Study the drawing (mm; zero at the part's minimum x, y, z) and answer. Coordinates: 2 decimals unless noted, no trailing zeros. Order: outer loops, then holes, each group sorted by start corner. A loop starts at its lowest first (then second) coordinate and runs counter-clockwise, first axis right, second up. Notation, with made-up numbers: M 71.25,82.5 L 93.25,82.5 A29 ccw 93.25,108.5 Z; hole C -33.5,12.5 d2. An arc over 180 degrees is marked long. Use a Markdown table: item, result. Add a question column.
1) Find the intervals of material crossed by probe 1 along Y at (x, z) = (85.5, 2); probe 2 along Y at (x, z) = (96, 1.8), in increasing order. Write a range as [from, to].
2) Find section B-B on z = 3.25. Count the separate pieces of the cut face and the enclosed holes in it, plus the area to 3 significant figures.
3) Find section A-A on x = 154. Write down the section's boundary in (y, z).
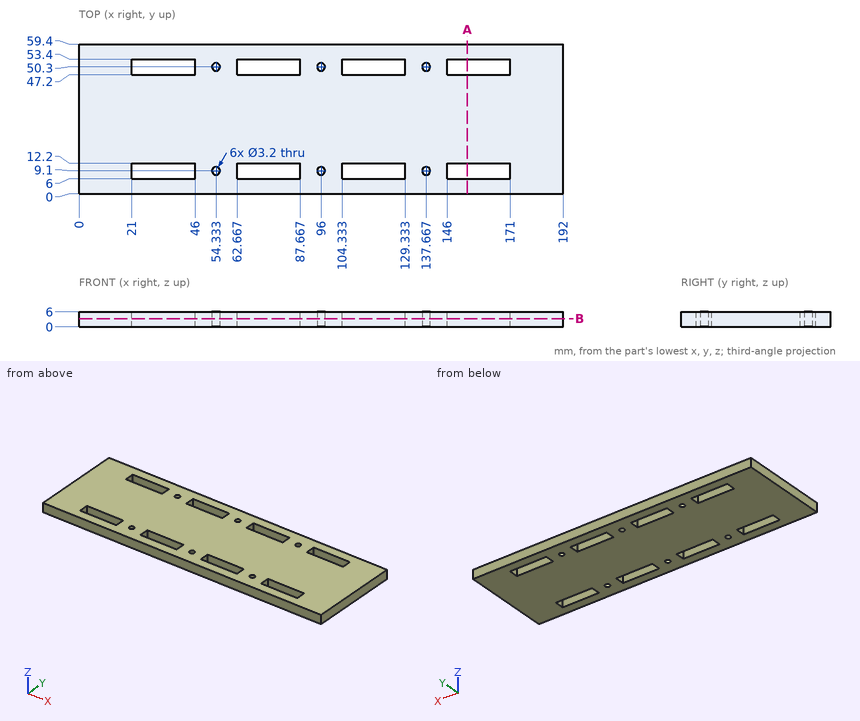
Check result:
| question | item | result |
|---|---|---|
| 1 | probe 1 | y = [0, 6], [12.2, 47.2], [53.4, 59.4] |
| 1 | probe 2 | y = [0, 7.5], [10.7, 48.7], [51.9, 59.4] |
| 2 | separate pieces | 1 |
| 2 | enclosed holes | 14 |
| 2 | area | 10,100 mm2 |
| 3 | outline | M 0,0 L 6,0 L 6,6 L 0,6 Z; M 12.2,0 L 47.2,0 L 47.2,6 L 12.2,6 Z; M 53.4,0 L 59.4,0 L 59.4,6 L 53.4,6 Z |
